Build history of the part. All positions in model axes, mm. A direction names the side the tool comes from. Round coordinates to 2 decimals unless told otherwise and drop trailing zeros. Write each loop counter-clockwise with the first axis right and the second up, starting at its lowest first coordinate (ties: lowest second). Pieces come first, ordered by that corner, then holes. Notation, with made-up numbers: (53.25, 30) - (65.25, 30) arc R23 cw to (65.25, 62) - close; hole circle Ø4 at (8.5, 43). An arc over 180 degrees is marked (long way). One line per question, with ' | ' between items.
from build123d import *

# Parameters (mm, degrees)
CROQUIS1_R              = 2.5
CROQUIS1_R_2            = 1.5
CROQUIS1_R_3            = 1.1
SALIENTE_EXTRUIR1_DEPTH = 3


with BuildPart() as part:
    # Croquis1 → Saliente-Extruir1 (new body)
    # profile 1 of 3: a face of its own
    with BuildSketch(Plane.XY):
        with BuildLine():
            ThreePointArc((-1.767766953, -1.767766953), (-1.767766953, 1.767766953), (1.767766953, 1.767766953))
            Line((1.767766953, 1.767766953), (-1, 4.535533906))
            Line((-1, 4.535533906), (-1, 20.464466094))
            Line((-1, 20.464466094), (1.767766953, 23.232233047))
            ThreePointArc((1.767766953, 23.232233047), (-1.767766953, 23.232233047), (-1.767766953, 26.767766953))
            Line((-1.767766953, 26.767766953), (-6, 22.535533906))
            Line((-6, 22.535533906), (-6, 2.464466094))
            Line((-6, 2.464466094), (-1.767766953, -1.767766953))
        make_face()
    # profile 2 of 3: a face of its own
    with BuildSketch(Plane.XY):
        with Locations((0, 25)):
            Circle(CROQUIS1_R)
        with Locations((0, 25)):
            Circle(CROQUIS1_R_2, mode=Mode.SUBTRACT)
    # profile 3 of 3: a face of its own
    with BuildSketch(Plane.XY):
        Circle(CROQUIS1_R)
        Circle(CROQUIS1_R_3, mode=Mode.SUBTRACT)
    extrude(amount=SALIENTE_EXTRUIR1_DEPTH)


solid = part.part
Q1. Pull direction X, two halves, no side cores. Call faces 1 (the cylindrical face through (-0.195, 26.487, 1.479)), 2 (the flat face through (-1, 12, 1)), 3 (the flat face through (-6, 13, 1)): +X half, -X half, draft (parallel to the pull), parting line (faces both ways), or undercut.
Found:
face 1: undercut | face 2: +X half | face 3: -X half
Q2. Saw through at A-A, the plane x = 0. List the corners of the cut face in (y, z), then the cut area to 3 significant figures.
Found:
outline: (-2.5, 0) - (-1.1, 0) - (-1.1, 3) - (-2.5, 3) - close; (1.1, 0) - (3.54, 0) - (3.54, 3) - (1.1, 3) - close; (21.46, 0) - (23.5, 0) - (23.5, 3) - (21.46, 3) - close; (26.5, 0) - (27.5, 0) - (27.5, 3) - (26.5, 3) - close | area: 20.6 mm^2
Q3. Saw through at B-B, the plane z = 1.15. List the corners of the cut face in (x, y).
Found:
outline: (-6, 2.46) - (-1.77, -1.77) arc R2.5 ccw to (1.77, 1.77) - (-1, 4.54) - (-1, 20.46) - (1.77, 23.23) arc R2.5 ccw to (-1.77, 26.77) - (-6, 22.54) - close; hole circle Ø3 at (0, 25); hole circle Ø2.2 at (0, 0)
Q4. Which spindle directions (+Z, -Z, +X, -X, +Y, -Y) get a long thin tool onto all of the face, cutting with end or side? Do faces 4 (the cylindrical face through (1.05, 0.33, 1.48)), 5 (the flat face through (0.403, 3.132, 1.479)). Say none if no direction does.
Found:
face 4: +Z, -Z | face 5: +Z, -Z, +X
Q5. Saw through at D-D, the plane y = 25. List the corners of the cut face in (x, z).
Found:
outline: (-3.54, 0) - (-1.5, 0) - (-1.5, 3) - (-3.54, 3) - close; (1.5, 0) - (2.5, 0) - (2.5, 3) - (1.5, 3) - close
Q6. Drop flat-ended pins along their axis: pin 1 (2 mm diameter, centred on x = 0, y = 0, fed in from +Z); pin 2 (1 mm diameter, centred on y = 13.5, z = 1.5, fed in from +X). Give the stop position or say it passes through.
Found:
pin 1: through | pin 2: x = -1
Q7. Saw through at C-C, the plane y = 0. List the corners of the cut face in (x, z).
Found:
outline: (-3.54, 0) - (-1.1, 0) - (-1.1, 3) - (-3.54, 3) - close; (1.1, 0) - (2.5, 0) - (2.5, 3) - (1.1, 3) - close
Q8. Drill centre lines: L1, parallel to Y at x = 0, z = 1.5; L2, parallel to Y at x = -0.25, z = 1.05; L3, parallel to X at y = 7.25, z = 0.4. Where is each one in solid material? Low to high. Write a range as from..to.
Found:
L1: -2.5..-1.1, 1.1..3.54, 21.46..23.5, 26.5..27.5 | L2: -2.49..-1.07, 1.07..3.79, 21.21..23.52, 26.48..27.49 | L3: -6..-1
